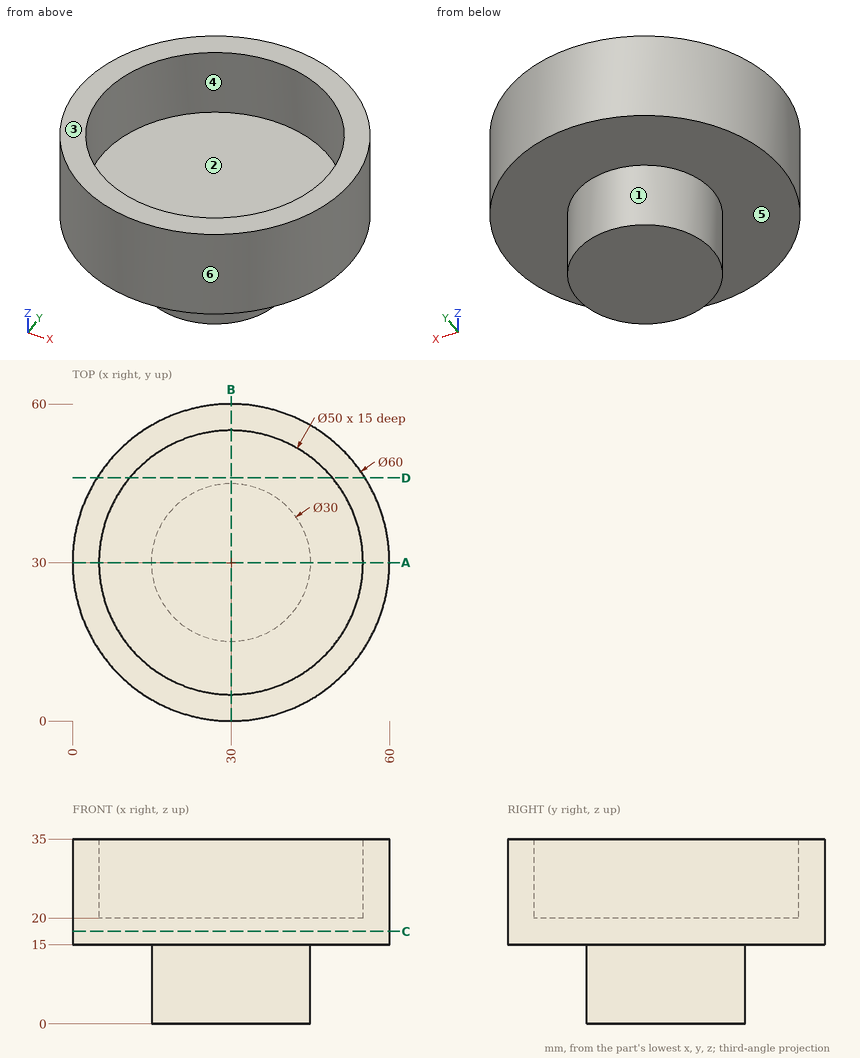
Geometry: see drawing. Coordinates: mm, zero at the bounding-box minimum. A direction names the side the tool comes from. Coordinates: 2 decimals unless noted, no trailing zeros. Loops run counter-clockwise (first coordinate to the right, second up) from the corner with the lowest first, then second, coordinate; pieces in that order, holes last. Notation, with made-up numbers: M 3.5,-9.5 L 54.5,-9.5 A31 ccw 54.5,18.5 Z; hole C 16.5,65.25 d1. An arc over 180 degrees is marked long. Put each result on its own line as item: value. Start each with the question number.
1) Cut plane C-C on z = 17.5. Return the cut outline in (x, y).
2) Contact query for flat-ended pins moving along their axis: pin 1 Ø15 at (x, y) = (29, 29.5) entering from +Z; pin 2 Ø4 at (x, z) = (9.5, 27.5) entering from +Y; pin 3 Ø10 at (x, y) = (6.5, 18) entering from -Z. Output: stop coordinate, or through.
3) Pull-direction query (X, two-part tool) for the marked faces 1, 2 and 3; classes: pulls with the +X half, pulls with the -X half, needs draft (parallel to the pull), parting line crosses it, or undercut.
4) Cut plane D-D on y = 46. Return the cut outline in (x, z), then the cut area to 3 significant figures.
5) Cut plane A-A on y = 30. Return the cut outline in (x, z).
6) Ray query, L1, parallel to Y at x = 30, z = 26.75; L2, parallel to Z at x = 7, y = 37.5; L3, parallel to X at y = 29, z = 15.5. Return the intervals inside material, ascending. Write a range as from..to.
7) Reachability of the marked faces 4, 5 and 6 from +Z, -Z, +X, -X, +Y, -Y: full face, straight path, thin tool, end or side. Return the list, or none.
The answers:
1. outline: C 30,30 d60
2. pin 1: stops at z = 20
2. pin 2: stops at y = 53.62
2. pin 3: stops at z = 15
3. face 1: parting line crosses it
3. face 2: undercut
3. face 3: needs draft
4. outline: M 4.62,15 L 55.38,15 L 55.38,35 L 49.21,35 L 49.21,20 L 10.79,20 L 10.79,35 L 4.62,35 Z
4. area: 439 mm²
5. outline: M 0,15 L 15,15 L 15,0 L 45,0 L 45,15 L 60,15 L 60,35 L 55,35 L 55,20 L 5,20 L 5,35 L 0,35 Z
6. L1: y = 0..5, 55..60
6. L2: z = 15..20
6. L3: x = 0.02..59.98
7. face 4: +Z
7. face 5: -Z
7. face 6: +Z, -Z
